CAD build for the part. Positions are in the model's coordinates, mm. A direction names the side the tool comes from. Coordinates: 2 decimals unless noted, no trailing zeros. Order: outer loops, then holes, each group sorted by start corner. A loop starts at its lowest first (then second) coordinate and runs counter-clockwise, first axis right, second up. Notation, with made-up numbers: M -11.5,51.25 L 10.5,51.25 A6 cw 10.5,56.25 Z; hole C 81,36.5 d1. An arc over 180 degrees is marked long. Write item = value, one per line.
from build123d import *

# Parameters (mm, degrees)
F0_R           = 2.75
F0_R_2         = 6
F1_DEPTH       = 10
F3_D           = 6.6
F3_CBORE_D     = 10.8
F3_CBORE_DEPTH = 1.5


with BuildPart() as f1:
    # F0 (on Front) → F1 (new body, symmetric)
    with BuildSketch(Plane.XZ):
        Polygon((-30, 7.5), (-30, -25), (30, -25), (30, 7.5), (17, 7.5), (17, 16), (15, 18), (-15, 18), (-17, 16), (-17, 7.5), align=None)
        with Locations((-23, -18)):
            Circle(F0_R, mode=Mode.SUBTRACT)
        with Locations((23, -18)):
            Circle(F0_R, mode=Mode.SUBTRACT)
        with Locations((-23, 0)):
            Circle(F0_R, mode=Mode.SUBTRACT)
        Circle(F0_R_2, mode=Mode.SUBTRACT)
        with Locations((23, 0)):
            Circle(F0_R, mode=Mode.SUBTRACT)
    extrude(amount=F1_DEPTH, both=True)

    # F3 (through all)
    with Locations(Plane.XY.offset(7.5)):
        with Locations((-23, 0), (23, 0)):
            CounterBoreHole(F3_D / 2, F3_CBORE_D / 2, F3_CBORE_DEPTH)


solid = f1.part
(1) Wall check: line 1 (Z direction, x = -23, y = 6.5); line 2 (X direction, y = -4.5, z = -18); line 3 (Y direction, x = 23, z = 6.85). Give the ranges that are in metal, low to high. Write a range as from..to.
Evaluation:
line_1 = -25..-20.75, -15.25..-2.75, 2.75..7.5
line_2 = -30..-25.75, -20.25..20.25, 25.75..30
line_3 = -10..-5.4, 5.4..10
(2) Slice it at D-D, the plane x = -23. Write the cut outline in (y, z), then the cut area to 3 significant figures.
Evaluation:
outline = M -10,-25 L -3.3,-25 L -3.3,-20.75 L -10,-20.75 Z; M -10,-15.25 L -3.3,-15.25 L -3.3,-2.75 L -10,-2.75 Z; M -10,2.75 L -3.3,2.75 L -3.3,6 L -5.4,6 L -5.4,7.5 L -10,7.5 Z; M 3.3,-25 L 10,-25 L 10,-20.75 L 3.3,-20.75 Z; M 3.3,-15.25 L 10,-15.25 L 10,-2.75 L 3.3,-2.75 Z; M 3.3,2.75 L 10,2.75 L 10,7.5 L 5.4,7.5 L 5.4,6 L 3.3,6 Z
area = 282 mm²
(3) Slice it at B-B, the plane x = 0. Write the cut outline in (y, z).
Evaluation:
outline = M -10,-25 L 10,-25 L 10,-6 L -10,-6 Z; M -10,6 L 10,6 L 10,18 L -10,18 Z
(4) Pull direction X, two halves, no side cores. Call faces 5 (the face through (0, 0, -25)), 6 (the face through (30, 0, -9)), 7 (the face through (25.62, -5.85, -17.17)): +X half, -X half, draft (parallel to the pull), parting line (faces both ways), or undercut.
Evaluation:
face_5 = draft
face_6 = +X half
face_7 = undercut
(5) Slice it at A-A, the plane y = 0. Write the cut outline in (x, z).
Evaluation:
outline = M -30,-25 L -26.3,-25 L -26.3,6 L -28.4,6 L -28.4,7.5 L -30,7.5 Z; M -19.7,-25 L 19.7,-25 L 19.7,6 L 17.6,6 L 17.6,7.5 L 17,7.5 L 17,16 L 15,18 L -15,18 L -17,16 L -17,7.5 L -17.6,7.5 L -17.6,6 L -19.7,6 Z; M 26.3,-25 L 30,-25 L 30,7.5 L 28.4,7.5 L 28.4,6 L 26.3,6 Z; hole C 0,0 d12
(6) Pin check, flat tips, straight feed: pin 1 Ø8.5 at (x, y) = (23, 0) entering from -Z; pin 2 Ø7 at (y, z) = (2, 13.5) entering from +X; pin 3 Ø5.5 at (x, y) = (-21, -1.5) entering from +Z; pin 4 Ø4 at (x, y) = (-23.5, 4.5) entering from +Z. Stop position of each tip, or through.
Evaluation:
pin_1 = -25
pin_2 = 17
pin_3 = 6
pin_4 = 7.5
(7) Slice it at C-C, the plane z = 0. Write the cut outline in (x, y), then the cut area to 3 significant figures.
Evaluation:
outline = M -30,-10 L -25.75,-10 L -25.75,-1.82 A3.3 cw -25.75,1.82 L -25.75,10 L -30,10 Z; M -20.25,-10 L -6,-10 L -6,10 L -20.25,10 L -20.25,1.82 A3.3 cw -20.25,-1.82 Z; M 6,-10 L 20.25,-10 L 20.25,-1.82 A3.3 cw 20.25,1.82 L 20.25,10 L 6,10 Z; M 25.75,-10 L 30,-10 L 30,10 L 25.75,10 L 25.75,1.82 A3.3 cw 25.75,-1.82 Z
area = 735 mm²
(8) Tool access for faces 1 (the face through (-26, -5, 7.5)), 2 (the face through (-17.85, 1.62, 6.76)), 3 (the face through (26, -5, 7.5)), 4 (the face through (-6, 0, 0)): list every direction of +Z, -Z, +X, -X, +Y, -Y with a clear straight run to the whole face (end or side of a thin tool).
Evaluation:
face_1 = +Z, -X, +Y, -Y
face_2 = +Z
face_3 = +Z, +X, +Y, -Y
face_4 = +Y, -Y
